```python
from build123d import *

# Parameters (mm, degrees)
BOSS_EXTRUDE2_DEPTH = 20
SKETCH2_R           = 5
BOSS_EXTRUDE3_DEPTH = 40
SKETCH8_R           = 4
CUT_EXTRUDE1_DEPTH  = 40


with BuildPart() as part:
    # Sketch1 → Boss-Extrude2 (new body)
    with BuildSketch(Plane.XY):
        with BuildLine():
            Line((-3.678627735, 14.541928964), (-3.678627735, 18.081928964))
            Line((-3.678627735, 18.081928964), (4.321372265, 18.081928964))
            Line((4.321372265, 18.081928964), (4, 14.456832295))
            ThreePointArc((4, 14.456832295), (-0.166223927, -14.999078959), (-3.678627735, 14.541928964))
        make_face()
    extrude(amount=BOSS_EXTRUDE2_DEPTH)

    # Sketch2 → Boss-Extrude3 (add)
    with BuildSketch(Plane.XY.offset(20)):
        Circle(SKETCH2_R)
    extrude(amount=BOSS_EXTRUDE3_DEPTH)

    # Sketch8 → Cut-Extrude1 (cut)
    with BuildSketch(Plane.XY.offset(60)):
        Circle(SKETCH8_R)
    extrude(amount=-CUT_EXTRUDE1_DEPTH, mode=Mode.SUBTRACT)


solid = part.part
```
Could you check a few things on this model? Use its own coordinates, in mm. A direction names the side the tool comes from. Coordinates: 2 decimals unless noted, no trailing zeros. Write each loop counter-clockwise with the first axis right and the second up, starting at its lowest first coordinate (ties: lowest second). Pieces come first, ordered by that corner, then holes. Notation, with made-up numbers: M -39.75,-20.5 L -27.75,-20.5 A28 ccw -27.75,-0.5 Z; hole C -29,68 d5. An arc over 180 degrees is marked long. Answer as CSV lines item,"result". Start each with the question number.
1) I want a section at A-A, the plane y = 0. Please give me the cut outline in (x, z).
2) I want a section at C-C, the plane x = 0. Please give me the cut outline in (y, z), and give its area (3 significant figures).
3) For faces 5 (the flat face through (0, 2, 0)), 6 (the cylindrical face through (-1.08, -4.88, 39.72)), 7 (the flat face through (4.163, 16.295, 9.86)), which set-ups out of +Z, -Z, +X, -X, +Y, -Y let a thin tool reach every point of the face, with its end or its side?
4) For P1, Ø4, axis at y = -2.5, z = 29, coming from the +X side; P2, Ø2, axis at y = -8.5, z = 17.5, coming from the -X side; P3, Ø5, axis at x = -11.5, y = -6.5, coming from the +Z side, each with a flat end and sliding along its axis, tell me the tip position at first contact or that it passes through.
5) I want a section at B-B, the plane z = 37. Please give me the cut outline in (x, y), and give its area (3 significant figures).
6) I want a section at D-D, the plane z = 11.5. Please give me the cut outline in (x, y).
7) Please list where these lines run through material, in increasing order: line 1 (Y direction, x = 0, z = 29); line 2 (Z direction, x = -5.5, y = 13); line 3 (X direction, y = 9.5, z = 12.5). Write a range as from..to.
8) We'd pull the mould along X, two halves only. Please class faces 1 (the flat face through (0, 18.082, 10)), 2 (the cylindrical face through (0, -15, 10)), 3 (the flat face through (-3.679, 16, 10)), 4 (the cylindrical face through (-0.867, -3.905, 40.28)): +X half, -X half, draft (parallel to the pull), parting line (faces both ways), or undercut.
Data:
1,outline,"M -15,0 L 15,0 L 15,20 L 5,20 L 5,60 L 4,60 L 4,20 L -4,20 L -4,60 L -5,60 L -5,20 L -15,20 Z"
2,outline,"M -15,0 L 18.08,0 L 18.08,20 L 5,20 L 5,60 L 4,60 L 4,20 L -4,20 L -4,60 L -5,60 L -5,20 L -15,20 Z"
2,area,"742 mm^2"
3,face 5,"-Z, +X, -X, +Y, -Y"
3,face 6,"+Z"
3,face 7,"+Z, -Z, +X"
4,P1,"stops at x = 4.97"
4,P2,"stops at x = -12.99"
4,P3,"stops at z = 20"
5,outline,"C 0,0 d10; hole C 0,0 d8"
5,area,"28.3 mm^2"
6,outline,"M -3.68,14.54 A15 ccw long 4,14.46 L 4.32,18.08 L -3.68,18.08 Z"
7,line 1,"y = -5..-4, 4..5"
7,line 2,"z = 0..20"
7,line 3,"x = -11.61..11.61"
8,face 1,"draft"
8,face 2,"parting line"
8,face 3,"-X half"
8,face 4,"undercut"
